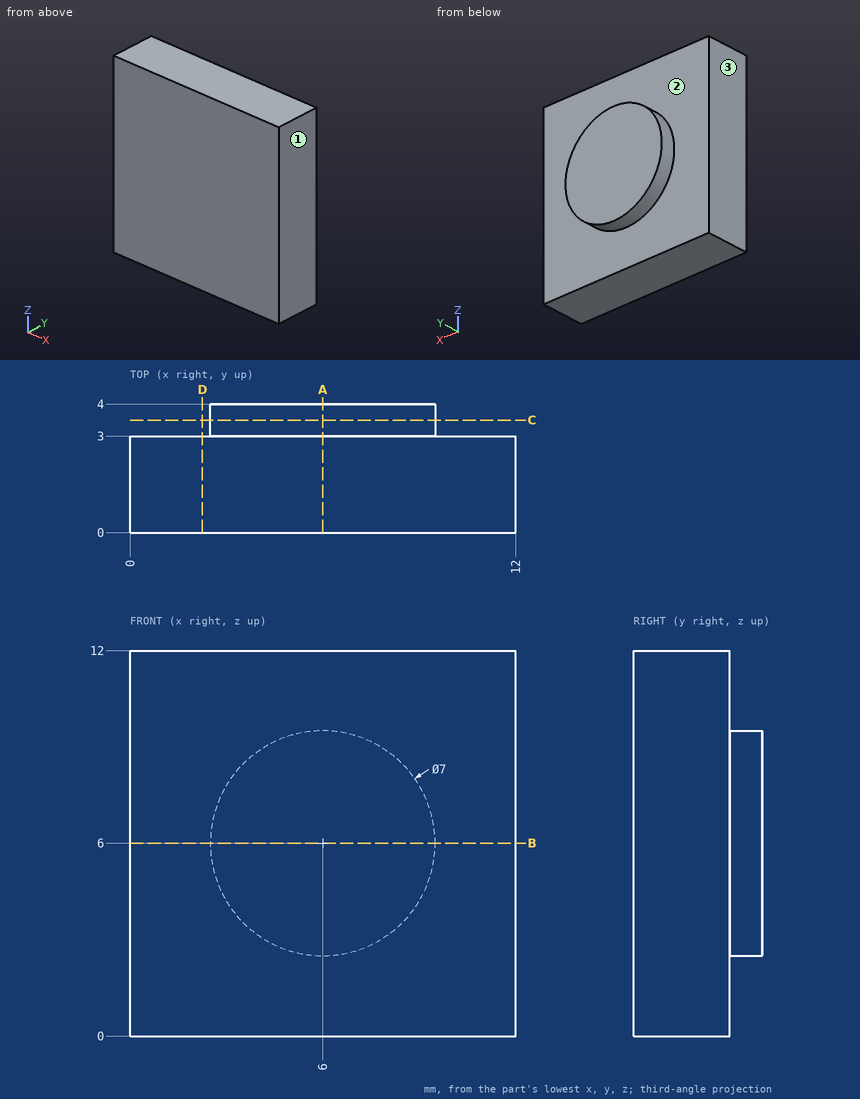
Input: dimensioned drawing with shaded views. Units: mm. Origin: part minimum x, y, z. Give positions to 0.01 mm unless a question says otherwise; leave off trailing zeros. Write each loop counter-clockwise with the first axis right and the second up, starting at its lowest first coordinate (ties: lowest second). Pieces come first, ordered by that corner, then holes. Notation, with made-up numbers: M 74.5,-14 L 85.5,-14 A23 cw 85.5,23 Z; hole C -30.5,-12 d1. An arc over 180 degrees is marked long. Return JSON: item names as keys, results as strings. Group by question number.
1) Material intervals for line 1 along Y through (x, z) = (4.75, 1.75); line 2 along X through (y, z) = (3.4, 3); line 3 along Z through (x, y) = (7.25, 3.6), sorted ascending. Write a range as [from, to].
2) Cut plane B-B, the plane z = 6. Output: boundary loops of the cut face in (x, y), plus the area to 3 significant figures.
3) Cut plane C-C, the plane y = 3.5. Output: boundary loops of the cut face in (x, z).
4) Pull-direction query (X, two-part tool) for the marked faces 1, 2 and 3; classes: pulls with the +X half, pulls with the -X half, needs draft (parallel to the pull), parting line crosses it, or undercut.
5) Cut plane A-A, the plane x = 6. Output: boundary loops of the cut face in (y, z), plus the area to 3 significant figures.
6) Cut plane D-D, the plane x = 2.25. Output: boundary loops of the cut face in (y, z).
Recorded:
{
 "1": {"line 1": "y = [0, 3]", "line 2": "x = [4.2, 7.8]", "line 3": "z = [2.73, 9.27]"},
 "2": {"outline": "M 0,0 L 12,0 L 12,3 L 9.5,3 L 9.5,4 L 2.5,4 L 2.5,3 L 0,3 Z", "area": "43.0 mm²"},
 "3": {"outline": "C 6,6 d7"},
 "4": {"face 1": "pulls with the +X half", "face 2": "needs draft", "face 3": "pulls with the -X half"},
 "5": {"outline": "M 0,0 L 3,0 L 3,2.5 L 4,2.5 L 4,9.5 L 3,9.5 L 3,12 L 0,12 Z", "area": "43.0 mm²"},
 "6": {"outline": "M 0,0 L 3,0 L 3,12 L 0,12 Z"}
}
